The model under review builds one solid part; all positions refer to its coordinate system, in mm. Face numbers are marked on the shaded views. A direction names the side the tool comes from. Coordinates: 2 decimals unless noted, no trailing zeros. Order: outer loops, then holes, each group sorted by start corner. A loop starts at its lowest first (then second) coordinate and runs counter-clockwise, first axis right, second up. Notation, with made-up numbers: (11, -13) -> (16, -13) arc R30 ccw to (16, 15) -> close; hole circle Ø8 at (43.5, 77.5). An arc over 180 degrees is marked (long way). Put each result on its own line as item: value.
from build123d import *

# Parameters (mm, degrees)
BOSS_EXTRUDE1_DEPTH         = 2.413
SKETCH2_W                   = 3.5687
SKETCH2_H                   = 0.762
F_1_4_20_TAPPED_HOLE1_D     = 5.1054
F_1_4_20_TAPPED_HOLE1_DEPTH = 16.51
F_1_4_20_TAPPED_HOLE1_TIP   = 1.533816902


with BuildPart() as part:
    # Sketch1 → Boss-Extrude1 (new body)
    with BuildSketch(Plane.XY.offset(2.413)):
        with BuildLine():
            Line((111.27866266, 120.306965896), (125.42646266, 120.306965896))
            ThreePointArc((125.42646266, 120.306965896), (131.05256266, 125.933065896), (125.42646266, 131.559165896))
            Line((125.42646266, 131.559165896), (111.27866266, 131.559165896))
            ThreePointArc((111.27866266, 131.559165896), (105.65256266, 125.933065896), (111.27866266, 120.306965896))
        make_face()
    extrude(amount=-BOSS_EXTRUDE1_DEPTH)

    # Sketch2 → Revolve1 (revolve)
    with BuildSketch(Plane.XZ.offset(-125.933065896), mode=Mode.PRIVATE) as revolve1_sk:
        with Locations((120.13691266, 2.794)):
            Rectangle(SKETCH2_W, SKETCH2_H)
    revolve(revolve1_sk.sketch.rotate(Axis((118.35256266, 125.933065896, 3.175), (0, 0, -1)), 180), axis=Axis((118.35256266, 125.933065896, 3.175), (0, 0, -1)))

    # 1/4-20 Tapped Hole1
    with Locations(Plane.XY.offset(3.175)):
        with Locations((118.35256266, 125.933065896)):
            Hole(F_1_4_20_TAPPED_HOLE1_D / 2, depth=F_1_4_20_TAPPED_HOLE1_DEPTH)
            with Locations((0, 0, -(F_1_4_20_TAPPED_HOLE1_DEPTH + F_1_4_20_TAPPED_HOLE1_TIP / 2))):  # 118° drill point
                Cone(0, F_1_4_20_TAPPED_HOLE1_D / 2, F_1_4_20_TAPPED_HOLE1_TIP, mode=Mode.SUBTRACT)


solid = part.part
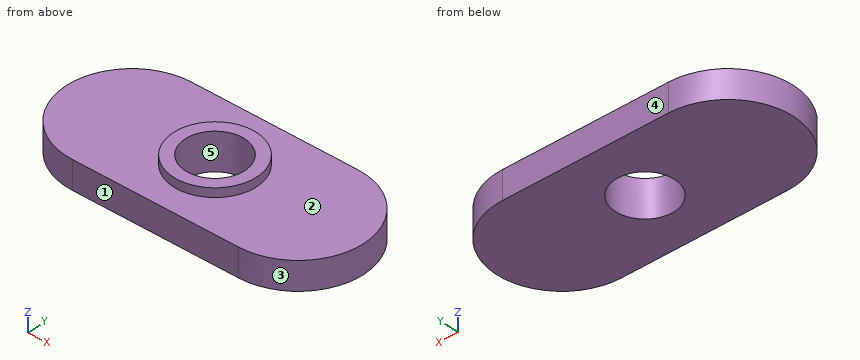
Item 1: Consider section B-B on x = 120. Write out the cut boundary in (y, z) (3 decimals), and give its area (3 significant figures).
Answers below:
outline: (120.307, 0) -> (123.983, 0) -> (123.983, 3.175) -> (122.767, 3.175) -> (122.767, 2.413) -> (120.307, 2.413) -> close; (127.883, 0) -> (131.559, 0) -> (131.559, 2.413) -> (129.099, 2.413) -> (129.099, 3.175) -> (127.883, 3.175) -> close
area: 19.6 mm^2
Item 2: For line 1 (X direction, y = 126, z = 1.9); line 2 (Z direction, x = 126.75, y = 126); line 3 (Y direction, x = 116.5, z = 1.35), list the stretches that pass through material, from the lowest coordinate up. Write a range as from..to.
Answers below:
line 1: 105.65..115.8, 120.9..131.05
line 2: 0..2.41
line 3: 120.31..124.18, 127.69..131.56
Item 3: For the marked faces 1 and 2, list the 3-axis set-ups (+Z, -Z, +X, -X, +Y, -Y) from which the entire face can be reached by the end or side of a thin tool; tool diameter is ignored.
Answers below:
face 1: +Z, -Z, +X, -X, -Y
face 2: +Z
Item 4: Consider section D-D on y = 128.75. Write out the cut boundary in (x, z) (3 decimals).
Answers below:
outline: (106.409, 0) -> (130.297, 0) -> (130.297, 2.413) -> (120.544, 2.413) -> (120.544, 3.175) -> (116.162, 3.175) -> (116.162, 2.413) -> (106.409, 2.413) -> close
Item 5: Consider section A-A on y = 125. Write out the cut boundary in (x, z) (1 decimal).
Answers below:
outline: (105.7, 0) -> (116, 0) -> (116, 3.2) -> (114.9, 3.2) -> (114.9, 2.4) -> (105.7, 2.4) -> close; (120.7, 0) -> (131, 0) -> (131, 2.4) -> (121.8, 2.4) -> (121.8, 3.2) -> (120.7, 3.2) -> close
Item 6: Mouldability with a two-part tool opening along X and no side actions: class the marked faces 3, 4 and 5 as +X half, -X half, draft (parallel to the pull), parting line (faces both ways), or undercut.
Answers below:
face 3: +X half
face 4: draft
face 5: undercut
